Autodesk Inventor part; units mm, degrees
ref_plane "YZ Plane" through (0, 0, 0) normal (1, 0, 0) x (0, 1, 0)
ref_plane "XZ Plane" through (0, 0, 0) normal (0, 1, 0) x (-1, 0, 0)
ref_plane "XY Plane" through (0, 0, 0) normal (0, 0, 1) x (1, 0, 0)
sketch "Sketch2" plane through (0, 0, 0) normal (0, 1, 0) x (-1, 0, 0)
  line L0 (0, 0) -> (-58, 0)
  line L1 (-58, 0) -> (-58, 85)
  line L2 (-58, 85) -> (0, 85)
  line L3 (0, 85) -> (0, 0)
  dimension "d0" = 58
  dimension "d1" = 85
extrude "Extrusion1" add sketch "Sketch2" along normal blind 20
shell "Shell1" thickness 3 removed faces 1 at (19.3333, 20, 28.3333)
sketch "Sketch4" plane through (58, 0, 0) normal (0, 0, -1) x (-1, 0, 0)
  point P0 (58, 0)
sketch "Sketch5" plane through (3, 3, 3) normal (0, 0, 1) x (1, 0, 0)
  line L0 (0, 0) -> (0, 17)
  line L1 (0, 17) -> (52, 17)
  line L2 (0, 0) -> (52, 0)
  line L3 (52, 0) -> (52, 17)
  line L4 (52, 17) -> (0, 17)
  line L5 (0, 17) -> (0, 0)
  point P0 (-3, -3)
extrude "Extrusion3" cut sketch "Sketch5" against normal blind 10
sketch "Sketch6" plane through (0, 0, 0) normal (-1, 0, 0) x (0, 0, 1)
  line L0 (4.5, 15.5) -> (30.5, 15.5)
  line L1 (30.5, 15.5) -> (30.5, 11.7)
  line L2 (30.5, 11.7) -> (4.5, 11.7)
  line L3 (4.5, 11.7) -> (4.5, 15.5)
  line L4 (0, 0) -> (0, 20)
  line L5 (0, 0) -> (85, 0)
  line L6 (0, 20) -> (85, 20)
  dimension "d19" = 26
  dimension "d20" = 3.8
  dimension "d21" = 4.5
  dimension "d34" = 11.7
sketch "Sketch7" plane through (58, 0, 85) normal (1, 0, 0) x (0, 0, -1)
  line L0 (0, 0) -> (85, 0)
  line L1 (0, 20) -> (85, 20)
  line L2 (85, 20) -> (85, 0)
  line L3 (85, 0) -> (0, 0)
  line L4 (0, 0) -> (0, 20)
extrude "Extrusion5" add sketch "Sketch7" along normal blind 3
extrude "Extrusion6" cut sketch "Sketch6" against normal through all
sketch "Sketch8" plane through (0, 0, 0) normal (-1, 0, 0) x (0, 0, 1)
  circle A0 centre (57.75, 15.5) radius 2.5
  line L0 (0, 20) -> (85, 20)
  line L1 (85, 0) -> (85, 20)
  line L2 (30.5, 15.5) -> (30.5, 11.7)
  point P0 (0, 0)
  point P1 (30.5, 13.6)
  dimension "d29" = 5
  dimension "d32" = 4.5
  dimension "d35" = 54.5
  dimension "d36" = 27.25
extrude "Extrusion7" cut sketch "Sketch8" against normal through all
equation "\"d36\" = 0.5 * d35"
properties part number "breadboard box v04"
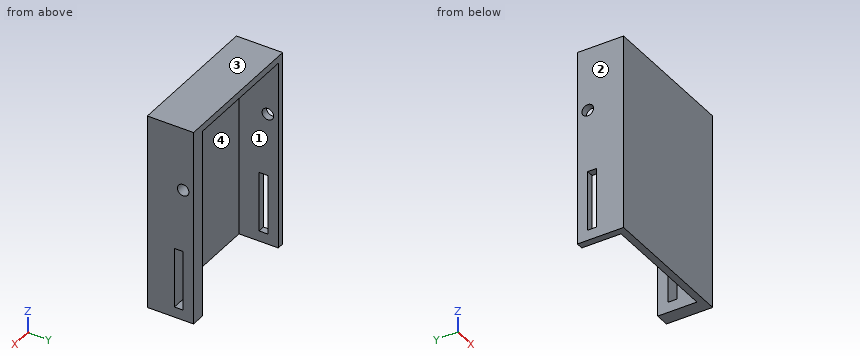
The listing builds one solid part. Answer for the finished solid, in the listing's coordinates (mm). Face numbers are marked on the shaded views. Coordinates: 2 decimals unless noted, no trailing zeros. Loops run counter-clockwise (first coordinate to the right, second up) from the corner with the lowest first, then second, coordinate; pieces in that order, holes last. Notation, with made-up numbers: M 45.25,86 L 59.25,86 A6 cw 59.25,93 Z; hole C 88.25,75.25 d3. An arc over 180 degrees is marked long. Answer as CSV lines item,"result". Start each with the question number.
(1) Find the intervals of material crossed by L1, parallel to X at y = 5.75, z = 10; L2, parallel to Y at x = 58.45, z = 57.75; L3, parallel to Z at x = 29, y = 8.5, in increasing order. Write a range as [from, to].
(2) The part is cut by section C-C (x = 56). Give the vertices of the cut face in (y, z), and give its area (3 significant figures).
(3) The part is cut by section D-D (z = 25.5). Give the vertices of the cut face in (x, y), and give its area (3 significant figures).
(4) The part is cut by section A-A (z = 57.75). Give the vertices of the cut face in (x, y), and give its area (3 significant figures).
(5) Given pin 1 (3 mm diameter, centred on x = 29, z = 12, fed in from +Y), flat-ended and moving along its own axis, determine where the tip first touches the part or whether it passes through.
(6) The part is cut by section B-B (y = 4.5). Give the vertices of the cut face in (x, z).
(7) The mould has two halves that part along X. Classify the marked faces 1, 2, 3 and 4: pulls with the +X half, pulls with the -X half, needs draft (parallel to the pull), parting line crosses it, or undercut.
Determined:
1,L1,"[0, 3], [55, 61]"
1,L2,"[0, 13], [18, 20]"
1,L3,"[82, 85]"
2,outline,"M 0,0 L 20,0 L 20,85 L 0,85 Z; hole M 11.7,4.5 L 15.5,4.5 L 15.5,30.5 L 11.7,30.5 Z; hole C 15.5,57.75 d5"
2,area,"1,580 mm2"
3,outline,"M 0,0 L 61,0 L 61,11.7 L 55,11.7 L 55,3 L 3,3 L 3,11.7 L 0,11.7 Z; M 0,15.5 L 3,15.5 L 3,20 L 0,20 Z; M 55,15.5 L 61,15.5 L 61,20 L 55,20 Z"
3,area,"302 mm2"
4,outline,"M 0,0 L 61,0 L 61,13 L 55,13 L 55,3 L 3,3 L 3,13 L 0,13 Z; M 0,18 L 3,18 L 3,20 L 0,20 Z; M 55,18 L 61,18 L 61,20 L 55,20 Z"
4,area,"291 mm2"
5,pin 1,"y = 3"
6,outline,"M 0,0 L 3,0 L 3,82 L 55,82 L 55,0 L 61,0 L 61,85 L 0,85 Z"
7,face 1,"undercut"
7,face 2,"pulls with the -X half"
7,face 3,"needs draft"
7,face 4,"undercut"
